Part model, mm, in its own coordinate system. Coordinates: 2 decimals unless noted, no trailing zeros. Order: outer loops, then holes, each group sorted by start corner. A loop starts at its lowest first (then second) coordinate and runs counter-clockwise, first axis right, second up.
```python
from build123d import *

# Parameters (mm, degrees)
SKETCH1_W           = 38.1
SKETCH1_H           = 25.4
BOSS_EXTRUDE1_DEPTH = 9.525
SKETCH2_R           = 1.5875
CUT_EXTRUDE1_DEPTH  = 47.770670564
FILLET1_R           = 2.54


with BuildPart() as part:
    # Sketch1 → Boss-Extrude1 (new body)
    with BuildSketch(Plane.XY):
        with Locations((19.05, 12.7)):
            Rectangle(SKETCH1_W, SKETCH1_H)
    extrude(amount=BOSS_EXTRUDE1_DEPTH)

    # Sketch2 → Cut-Extrude1 (cut, through all)
    with BuildSketch(Plane.XZ):
        with Locations(Location((6.35, 4.7625, 0), (0, 0, 270))):
            Circle(SKETCH2_R)
        with Locations(Location((31.75, 4.7625, 0), (0, 0, 90))):
            Circle(SKETCH2_R)
    extrude(amount=-CUT_EXTRUDE1_DEPTH, mode=Mode.SUBTRACT)

    # Fillet1
    fillet1_edges = [part.edges().sort_by_distance(p)[0] for p in [
        (38.1, 12.7, 0),
    ]]
    fillet(fillet1_edges, radius=FILLET1_R)


solid = part.part
```
(1) Slice it at A-A, the plane y = 12. State how many separate pieces and enclosed holes the cut face has, then the cut area to 3 significant figures.
(2) Pull direction X, two halves, no side cores. Call faces 1 (the face through (37.336, 12.878, 0.724)), 2 (the face through (0, 13, 5)), 3 (the face through (5.38, 12.52, 6.02)): +X half, -X half, draft (parallel to the pull), parting line (faces both ways), or undercut.
(3) Probe line 1 (Z direction, x = 31.75, y = 12) (3 decimals); line 2 (X direction, y = 23.5, z = 3.5); line 3 (X direction, y = 2.5, z = 4). List the from-to ranges inside material, lowest first.
(4) Slice it at B-B, the plane x = 31.75. Give the cut face in (y, z) (3 decimals).
Here are the results:
1. separate pieces: 1
1. enclosed holes: 2
1. area: 346 mm2
2. face 1: +X half
2. face 2: -X half
2. face 3: undercut
3. line 1: z = 0 to 3.175, 6.35 to 9.525
3. line 2: x = 0 to 5.39, 7.31 to 30.79, 32.71 to 38.1
3. line 3: x = 0 to 4.96, 7.74 to 30.36, 33.14 to 38.1
4. outline: (0, 0) - (25.4, 0) - (25.4, 3.175) - (0, 3.175) - close; (0, 6.35) - (25.4, 6.35) - (25.4, 9.525) - (0, 9.525) - close
